Geometry: see drawing. Coordinates: mm, zero at the bounding-box minimum. Coordinates: 2 decimals unless noted, no trailing zeros. Loops run counter-clockwise (first coordinate to the right, second up) from the corner with the lowest first, then second, coordinate; pieces in that order, holes last. Notation, with made-up numbers: (4, 1.5) -> (50, 1.5) arc R12 ccw to (50, 8.5) -> close; hole circle Ø10 at (-35, 46.25). An arc over 180 degrees is marked (long way). One line per item, written item: value. Start each with the question number.
Item 1: Contact query for flat-ended pins moving along their axis: pin 1 Ø1.5 at (x, z) = (413.5, 23.5) entering from -Y; pin 2 Ø4 at (x, y) = (426, 19.5) entering from -Z. Output: stop coordinate, or through.
Item 2: Section query B-B on x = 347. Return loops of the section in (y, z), then the cut area to 3 significant figures.
Item 3: Ray query, probe 1 along Y at (x, z) = (84, 43.5). Return the intervals inside material, ascending. Write a range as from..to.
Item 4: Section query A-A on z = 179. Return loops of the section in (x, y).
Item 5: Section query D-D on z = 131.5. Return loops of the section in (x, y).
Item 6: Section query C-C on x = 650. Return loops of the section in (y, z).
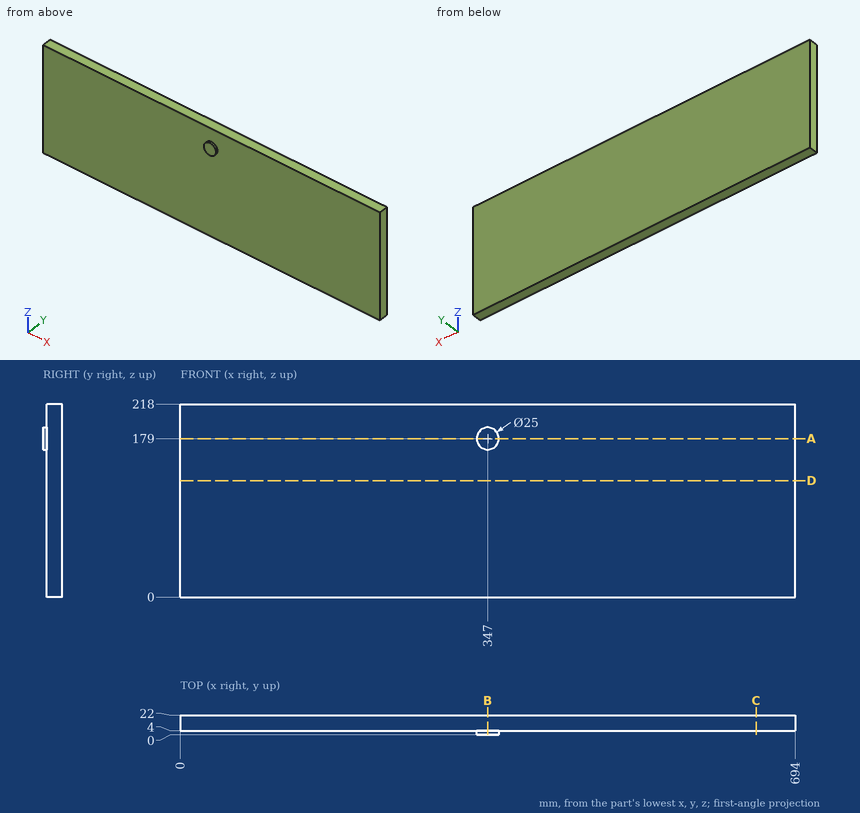
Reply:
1. pin 1: stops at y = 4
1. pin 2: stops at z = 0
2. outline: (0, 166.5) -> (4, 166.5) -> (4, 0) -> (22, 0) -> (22, 218) -> (4, 218) -> (4, 191.5) -> (0, 191.5) -> close
2. area: 4,020 mm²
3. probe 1: y = 4..22
4. outline: (0, 4) -> (334.5, 4) -> (334.5, 0) -> (359.5, 0) -> (359.5, 4) -> (694, 4) -> (694, 22) -> (0, 22) -> close
5. outline: (0, 4) -> (694, 4) -> (694, 22) -> (0, 22) -> close
6. outline: (4, 0) -> (22, 0) -> (22, 218) -> (4, 218) -> close
